```python
from build123d import *

# Parameters (mm, degrees)
EXTRUDE_1_DEPTH = 1.6
SKETCH_2_R      = 17.5
EXTRUDE_2_DEPTH = 2
SKETCH_3_W      = 50
SKETCH_3_H      = 40
EXTRUDE_3_DEPTH = 8.4
EXTRUDE_4_DEPTH = 5.3
SKETCH_5_W      = 2.9
SKETCH_5_H      = 2
EXTRUDE_5_DEPTH = 1.5
CHAMFER_1_SIZE  = 1


with BuildPart() as part:
    # 草图1 → 凸台-拉伸1 (new body)
    with BuildSketch(Plane.XY):
        Polygon((21.95697074, 22.538726334), (24.95697074, 19.538726334), (24.95697074, -22.461273666), (-25.04302926, -22.461273666), (-25.04302926, 22.538726334), align=None)
    extrude(amount=-EXTRUDE_1_DEPTH)

    # 草图2 → 凸台-拉伸2 (add)
    with BuildSketch(Plane.XY):
        Circle(SKETCH_2_R)
    extrude(amount=EXTRUDE_2_DEPTH)

    # 草图3 → 凸台-拉伸3 (add)
    with BuildSketch(Plane(origin=(0, 0, -1.6), x_dir=(-1, 0, 0), z_dir=(0, 0, -1))):
        with Locations((0.04302926, 2.538726334)):
            Rectangle(SKETCH_3_W, SKETCH_3_H)
    extrude(amount=EXTRUDE_3_DEPTH)

    # 草图4 → 凸台-拉伸4 (add)
    with BuildSketch(Plane.XZ.offset(17.461273666)):
        with BuildLine():
            Line((-2.9, -3.3), (2.9, -3.3))
            ThreePointArc((2.9, -3.3), (4.5, -4.9), (2.9, -6.5))
            Line((2.9, -6.5), (-2.9, -6.5))
            ThreePointArc((-2.9, -6.5), (-4.5, -4.9), (-2.9, -3.3))
        make_face()
    extrude(amount=EXTRUDE_4_DEPTH)

    # 草图5 → 凸台-拉伸5 (add)
    with BuildSketch(Plane(origin=(0, 0, -1.6), x_dir=(-1, 0, 0), z_dir=(0, 0, -1))):
        with Locations((16.99302926, -22.461273666)):
            Rectangle(SKETCH_5_W, SKETCH_5_H)
    extrude(amount=EXTRUDE_5_DEPTH)

    # 倒角1
    chamfer_1_edges = [part.edges().sort_by_distance(p)[0] for p in [
        (24.95697074, 22.538726334, -5.8),
        (-25.04302926, 22.538726334, -5),
        (24.95697074, -22.461273666, -0.8),
        (-25.04302926, -22.461273666, -0.8),
    ]]
    chamfer(chamfer_1_edges, length=CHAMFER_1_SIZE)


solid = part.part
```
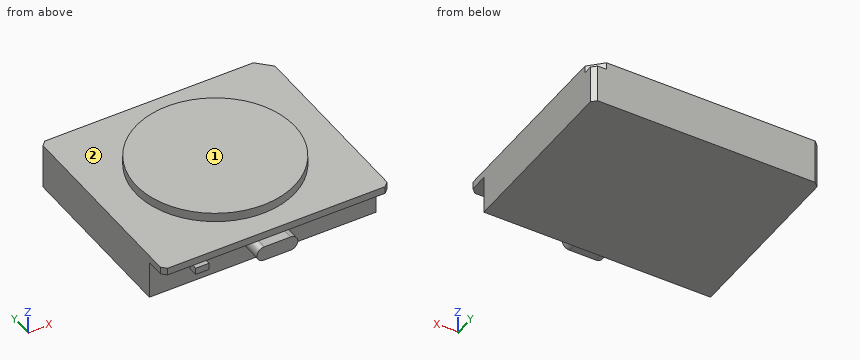
Geometry check sheet. Reference: the model listing, model coordinates, mm. Face numbers are marked on the shaded views. A direction names the side the tool comes from. Round coordinates to 2 decimals unless told otherwise and drop trailing zeros. Write each loop counter-clockwise with the first axis right and the second up, starting at its lowest first coordinate (ties: lowest second). Pieces come first, ordered by that corner, then holes. Notation, with made-up numbers: (81.25, 39) -> (121.25, 39) arc R10 cw to (121.25, 51) -> close; hole circle Ø10 at (74, -9). An arc over 180 degrees is marked (long way). Put each result on its own line as item: value.
1) Depth check by flat-ended pin: P1, Ø0.9, axis at x = 23.5, y = 21.5, coming from the +Z side; P2, Ø5.5, axis at x = 3, y = -20.5, coming from the -Z side; P3, Ø1, axis at x = 17, z = -1.5, coming from the -Y side. Enter the tip coordinate at first touch or a pass-through.
Recorded:
P1: stops at z = 0
P2: stops at z = -6.5
P3: stops at y = -22.46
2) Cross-section at A-A, the plane x = 0. Enter the section's corners in (y, z), plus the area to 3 significant figures.
Recorded:
outline: (-22.76, -6.5) -> (-17.46, -6.5) -> (-17.46, -10) -> (22.54, -10) -> (22.54, 0) -> (17.5, 0) -> (17.5, 2) -> (-17.5, 2) -> (-17.5, 0) -> (-22.46, 0) -> (-22.46, -1.6) -> (-17.46, -1.6) -> (-17.46, -3.3) -> (-22.76, -3.3) -> close
area: 495 mm2
3) Thickness scan on probe 1 along Y at (x, z) = (-2.5, -1); probe 2 along Y at (x, z) = (6, -5.5); probe 3 along Z at (x, y) = (10, 20.5). Record the ranges inside material, lowest first. Write a range as from..to.
Recorded:
probe 1: y = -22.46..22.54
probe 2: y = -17.46..22.54
probe 3: z = -10..0
4) Cross-section at D-D, the plane y = 9. Enter the section's corners in (x, z).
Recorded:
outline: (-25.04, -10) -> (24.96, -10) -> (24.96, 0) -> (15.01, 0) -> (15.01, 2) -> (-15.01, 2) -> (-15.01, 0) -> (-25.04, 0) -> close
5) Cross-section at B-B, the plane y = 0. Enter the section's corners in (x, z), plus the area to 3 significant figures.
Recorded:
outline: (-25.04, -10) -> (24.96, -10) -> (24.96, 0) -> (17.5, 0) -> (17.5, 2) -> (-17.5, 2) -> (-17.5, 0) -> (-25.04, 0) -> close
area: 570 mm2
6) Access from +Z, -Z, +X, -X, +Y, -Y to the whole of each face (thin tool, end or side, straight path). Record for the marked faces 1 and 2.
Recorded:
face 1: +Z, +X, -X, +Y, -Y
face 2: +Z
7) Cross-section at C-C, the plane z = -4.9. Enter the section's corners in (x, y).
Recorded:
outline: (-25.04, -17.46) -> (-4.5, -17.46) -> (-4.5, -22.76) -> (4.5, -22.76) -> (4.5, -17.46) -> (24.96, -17.46) -> (24.96, 21.54) -> (23.96, 22.54) -> (-24.04, 22.54) -> (-25.04, 21.54) -> close
